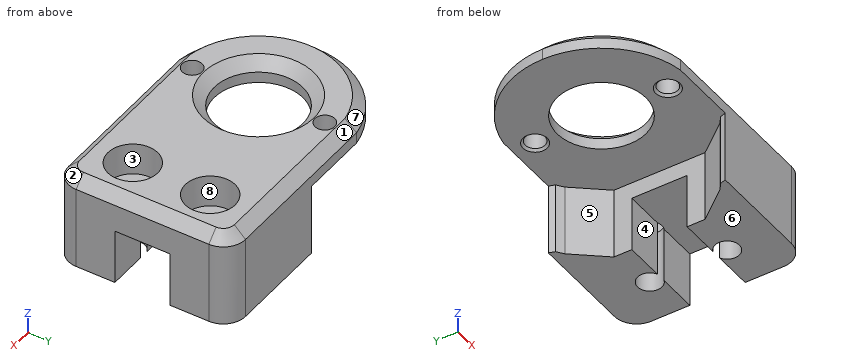
```python
from build123d import *

# Parameters (mm, degrees)
CROQUIS1_R              = 0.9
CROQUIS1_R_2            = 1.1
SALIENTE_EXTRUIR1_DEPTH = 8.5
REDONDEO1_R             = 2
CORTAR_EXTRUIR6_DEPTH   = 6.5
CHAFL_N1_SIZE           = 1
CHAFL_N1_SIZE_2         = 0.742384029
CROQUIS5_W              = 8
CROQUIS5_H              = 2.5
CORTAR_EXTRUIR7_DEPTH   = 5
CROQUIS6_R              = 2.25
CORTAR_EXTRUIR8_DEPTH   = 2.9
CHAFL_N3_SIZE           = 0.2
CROQUIS7_R              = 4
CORTAR_EXTRUIR9_DEPTH   = 20.80530232
CHAFL_N2_SIZE           = 1


with BuildPart() as part:
    # Croquis1 → Saliente-Extruir1 (new body)
    with BuildSketch(Plane.XY):
        with BuildLine():
            Line((-1.326649916, 8), (16, 8))
            Line((16, 8), (16, 0))
            Line((16, 0), (8, 0))
            Line((8, 0), (-8.109253973, 0))
            ThreePointArc((-8.109253973, 0), (-6.185391706, 5.24413286), (-1.326649916, 8))
        make_face()
        with Locations((0, 6)):
            Circle(CROQUIS1_R, mode=Mode.SUBTRACT)
        with Locations((12, 3.5)):
            Circle(CROQUIS1_R_2, mode=Mode.SUBTRACT)
    extrude(amount=SALIENTE_EXTRUIR1_DEPTH)

    # Redondeo1
    redondeo1_edges = [part.edges().sort_by_distance(p)[0] for p in [
        (16, 8, 4.25),
    ]]
    fillet(redondeo1_edges, radius=REDONDEO1_R)

    # Croquis4 → Cortar-Extruir6 (cut)
    with BuildSketch(Plane(origin=(0, 0, 0), x_dir=(-1, 0, 0), z_dir=(0, 0, -1))):
        with BuildLine():
            Line((-5.656854249, 7), (-8, 4.123105626))
            Line((-8, 4.123105626), (-8, 0))
            Line((-8, 0), (8.109253973, 0))
            Line((8.109253973, 0), (9, 0))
            ThreePointArc((9, 0), (3.878679656, 8.121320344), (-5.656854249, 7))
        make_face()
    extrude(amount=-CORTAR_EXTRUIR6_DEPTH, mode=Mode.SUBTRACT)

    # Chaflán1
    # the kernel refuses this chamfer: 1, 0.742384029 mm, written as the material it takes off along each edge
    with BuildSketch(Plane(origin=(16, 6, 8.5), x_dir=(-1, 0, 0), z_dir=(0, -1, 0))) as chafl_n1_piece_1:
        Polygon((CHAFL_N1_SIZE, 0), (0, CHAFL_N1_SIZE), (0, 0), align=None)
    extrude(amount=8.571682988, mode=Mode.SUBTRACT)
    with BuildSketch(Plane(origin=(-5.698510996, 8, 8.5), x_dir=(0, 0, -1), z_dir=(1, 0, 0))) as chafl_n1_piece_2:
        Polygon((CHAFL_N1_SIZE, 0), (0, -CHAFL_N1_SIZE), (0, 0), align=None)
    extrude(amount=19.698510996, mode=Mode.SUBTRACT)
    with BuildSketch(Plane(origin=(14, 6, 8.5), x_dir=(0, 1, 0), z_dir=(-1, 0, 0))) as chafl_n1_piece_3:
        Polygon((2, CHAFL_N1_SIZE), (2 - CHAFL_N1_SIZE, 0), (2, 0), align=None)
    revolve(axis=Axis((14, 6, 8.5), (0, 0, -1)), revolution_arc=90, mode=Mode.SUBTRACT)
    with BuildSketch(Plane(origin=(0, 0, 8.5), x_dir=(-0.9501026430594787, -0.3119374418876211, 0), z_dir=(0.3119374418876211, -0.9501026430594787, 0))) as chafl_n1_piece_4:
        Polygon((8.109253973 - CHAFL_N1_SIZE, 0), (8.109253973, CHAFL_N1_SIZE), (8.109253973, 0), align=None)
    revolve(axis=Axis((0, 0, 8.5), (0, 0, -1)), revolution_arc=116.936314038, mode=Mode.SUBTRACT)
    with BuildSketch(Plane(origin=(4.123105626, 8, 6.5), x_dir=(1, 0, 0), z_dir=(0, 0, -1))) as chafl_n1_piece_5:
        with BuildLine():
            Line((CHAFL_N1_SIZE_2, 0), (0.916025454, 0.542979283))
            ThreePointArc((0.916025454, 0.542979283), (0.478949419, 0.265590562), (0, 0))
            Line((0, 0), (CHAFL_N1_SIZE_2, 0))
        make_face()
    extrude(amount=9.23772815, mode=Mode.SUBTRACT)

    # Croquis5 → Cortar-Extruir7 (cut)
    with BuildSketch(Plane(origin=(0, 0, 0), x_dir=(-1, 0, 0), z_dir=(0, 0, -1))):
        with Locations((-12, 1.25)):
            Rectangle(CROQUIS5_W, CROQUIS5_H)
    extrude(amount=-CORTAR_EXTRUIR7_DEPTH, mode=Mode.SUBTRACT)

    # Croquis6 → Cortar-Extruir8 (cut)
    with BuildSketch(Plane.XY.offset(8.5)):
        with Locations((12, 3.5)):
            Circle(CROQUIS6_R)
    extrude(amount=-CORTAR_EXTRUIR8_DEPTH, mode=Mode.SUBTRACT)

    # Chaflán3
    chafl_n3_edges = [part.edges().sort_by_distance(p)[0] for p in [
        (-0.9, 6, 6.5),
    ]]
    chamfer(chafl_n3_edges, length=CHAFL_N3_SIZE)

    # Simetría1: part across plane


with BuildPart() as part_1:
    add(part.part)
    add(part.part.mirror(Plane(origin=(16, 0, 8.5), x_dir=(0, 0, 1), z_dir=(0, 1, 0))))

    # Croquis7 → Cortar-Extruir9 (cut, through all)
    with BuildSketch(Plane.XY.offset(8.5)):
        Circle(CROQUIS7_R)
    extrude(amount=-CORTAR_EXTRUIR9_DEPTH, mode=Mode.SUBTRACT)

    # Chaflán2
    chafl_n2_edges = [part_1.edges().sort_by_distance(p)[0] for p in [
        (-4, 0, 8.5),
    ]]
    chamfer(chafl_n2_edges, length=CHAFL_N2_SIZE)


solid = part_1.part
```
Geometry check sheet. Reference: the model listing, model coordinates, mm. Face numbers are marked on the shaded views. A direction names the side the tool comes from. Coordinates: 2 decimals unless noted, no trailing zeros. Loops run counter-clockwise (first coordinate to the right, second up) from the corner with the lowest first, then second, coordinate; pieces in that order, holes last.
Item 1: Go/stop test with flat-tipped pins: pin 1 Ø3.5 at (x, y) = (12, -3.5) entering from -Z; pin 2 Ø3 at (y, z) = (3, 5.5) entering from -X; pin 3 Ø2.5 at (x, y) = (12.5, 0) entering from -Z; pin 4 Ø5 at (x, z) = (-4, 4.5) entering from +Y. Record where each tip stops, or that it passes through.
Item 2: Sectioned sample at D-D, the plane z = 5.25. Record the boundary of the cut face in (x, y), then the cut area to 3 significant figures.
Item 3: Thickness scan on line 1 (Y direction, x = 0, z = 7.1); line 2 (Y direction, x = 12, z = 7.8); line 3 (X direction, y = -3.5, z = 2.95). Record the ranges inside material, lowest first.
Item 4: Sectioned sample at B-B, the plane z = 4. Record the boundary of the cut face in (x, y), then the cut area to 3 significant figures.
Item 5: Sectioned sample at C-C, the plane x = 12. Record the boundary of the cut face in (y, z).
Item 6: Sectioned sample at A-A, the plane x = 0. Record the boundary of the cut face in (y, z).
Item 7: Access from +Z, -Z, +X, -X, +Y, -Y to the whole of each face (thin tool, end or side, straight path). Record for the marked faces 4, 5, 6, 7 and 8.
Item 8: Release check for a two-part mould opening along Y. For the marked faces 1, 2 and 3 record: released by +Y, released by -Y, zero draft, split by the parting line, or undercut.
Check result:
1. pin 1: stops at z = 0
1. pin 2: stops at x = -7.89
1. pin 3: stops at z = 5
1. pin 4: stops at y = 7.71
2. outline: (4.87, -8) - (14, -8) arc R2 ccw to (16, -6) - (16, 6) arc R2 ccw to (14, 8) - (4.87, 8) - (5.04, 7.46) arc R9 cw to (5.66, 7) - (8, 4.12) - (8, -4.12) - (5.66, -7) arc R9 cw to (5.04, -7.46) - close; hole circle Ø2.2 at (12, -3.5); hole circle Ø2.2 at (12, 3.5)
2. area: 131 mm2
3. line 1: y = -8 to -6.9, -5.1 to -4, 4 to 5.1, 6.9 to 8
3. line 2: y = -7.7 to -5.75, -1.25 to 1.25, 5.75 to 7.7
3. line 3: x = 8 to 10.9, 13.1 to 16
4. outline: (4.87, -8) - (14, -8) arc R2 ccw to (16, -6) - (16, -2.5) - (12.46, -2.5) arc R1.1 cw (long way) to (11.54, -2.5) - (8, -2.5) - (8, -4.12) - (5.66, -7) arc R9 cw to (5.04, -7.46) - close; (4.87, 8) - (5.04, 7.46) arc R9 cw to (5.66, 7) - (8, 4.12) - (8, 2.5) - (11.54, 2.5) arc R1.1 cw (long way) to (12.46, 2.5) - (16, 2.5) - (16, 6) arc R2 ccw to (14, 8) - close
4. area: 91.3 mm2
5. outline: (-8, 0) - (-4.6, 0) - (-4.6, 5.6) - (-5.75, 5.6) - (-5.75, 8.5) - (-7, 8.5) - (-8, 7.5) - close; (-2.4, 5) - (2.4, 5) - (2.4, 5.6) - (1.25, 5.6) - (1.25, 8.5) - (-1.25, 8.5) - (-1.25, 5.6) - (-2.4, 5.6) - close; (4.6, 0) - (8, 0) - (8, 7.5) - (7, 8.5) - (5.75, 8.5) - (5.75, 5.6) - (4.6, 5.6) - close
6. outline: (-8, 6.5) - (-7.1, 6.5) - (-6.9, 6.7) - (-6.9, 8.5) - (-7, 8.5) - (-8, 7.5) - close; (-5.1, 6.7) - (-4.9, 6.5) - (-4, 6.5) - (-4, 7.5) - (-5, 8.5) - (-5.1, 8.5) - close; (4, 6.5) - (4.9, 6.5) - (5.1, 6.7) - (5.1, 8.5) - (5, 8.5) - (4, 7.5) - close; (6.9, 6.7) - (7.1, 6.5) - (8, 6.5) - (8, 7.5) - (7, 8.5) - (6.9, 8.5) - close
7. face 4: -Z, +X, -X
7. face 5: -Z, -X
7. face 6: -Z, +X, -X, +Y, -Y
7. face 7: +Z, -X
7. face 8: +Z
8. face 1: released by +Y
8. face 2: released by -Y
8. face 3: undercut
